Source: CAD feature listing. Evaluate the final solid. Frame: model axes, mm. Face numbers are marked on the shaded views. A direction names the side the tool comes from. Round coordinates to 2 decimals unless told otherwise and drop trailing zeros. Order: outer loops, then holes, each group sorted by start corner. A loop starts at its lowest first (then second) coordinate and runs counter-clockwise, first axis right, second up. Notation, with made-up numbers: (45.25, 1.25) -> (61.25, 1.25) arc R23 cw to (61.25, 14.25) -> close; hole circle Ø6 at (54.5, 48.25). An arc over 180 degrees is marked (long way). Answer as CSV lines item,"result".
Autodesk Fusion 360 part; units mm, degrees
sketch "Sketch1" plane through (0, 0, 0) normal (0, 0, 1) x (1, 0, 0)
  line L0 (-125, 90) -> (125, 90)
  line L1 (125, 90) -> (125, -90)
  line L2 (125, -90) -> (-125, -90)
  line L3 (-125, -90) -> (-125, 90)
  dimension "d1" = 250
  dimension "d2" = 180
  dimension "d3" = 90
  dimension "d4" = 125
extrude "Extrude1" add sketch "Sketch1" along normal blind 60
shell "Shell1" thickness 3 removed faces 1 at (-41.6667, 30, 60)
sketch "Sketch2" plane through (0, -90, 0) normal (0, -1, 0) x (1, 0, 0)
  line L0 (-125, 0) -> (125, 0)
  line L1 (125, 0) -> (125, 60)
  line L2 (125, 60) -> (-125, 60)
  line L3 (-125, 60) -> (-125, 0)
  circle A0 centre (-85, 30) radius 5
  circle A1 centre (25, 30) radius 5
  line L4 (-40, 35) -> (-10, 35)
  line L5 (-10, 35) -> (-10, 25)
  line L6 (-10, 25) -> (-40, 25)
  line L7 (-40, 25) -> (-40, 35)
  circle A2 centre (-110, 30) radius 6
  dimension "d8" = 10
  dimension "d9" = 10
  dimension "d10" = 12
extrude "Extrude2" cut sketch "Sketch2" against normal blind 10 contours A0 | A1 | L4 L5 L6 L7 | A2
sketch "Sketch3" plane through (0, 90, 0) normal (0, 1, 0) x (-1, 0, 0)
  line L0 (-125, 0) -> (125, 0)
  line L1 (125, 0) -> (125, 60)
  line L2 (125, 60) -> (-125, 60)
  line L3 (-125, 60) -> (-125, 0)
  circle A0 centre (105, 40) radius 5
  circle A1 centre (105, 25) radius 5
  circle A2 centre (90, 25) radius 5
  circle A3 centre (90, 40) radius 5
  circle A4 centre (105, 25) radius 5
  circle A5 centre (60, 25) radius 5
  circle A6 centre (75, 25) radius 5
  circle A7 centre (75, 25) radius 5
  circle A8 centre (75, 40) radius 5
  circle A9 centre (60, 40) radius 5
  line L4 (35, 45) -> (45, 45)
  line L5 (45, 45) -> (45, 30)
  line L6 (45, 30) -> (35, 30)
  line L7 (35, 30) -> (35, 45)
  line L8 (-110, 49) -> (-75, 49)
  line L9 (-75, 49) -> (-75, 14)
  line L10 (-75, 14) -> (-110, 14)
  line L11 (-110, 14) -> (-110, 49)
  dimension "d13" = 10
  dimension "d14" = 10
  dimension "d15" = 10
  dimension "d16" = 10
  dimension "d17" = 10
  dimension "d18" = 10
  dimension "d19" = 10
  dimension "d20" = 10
  dimension "d21" = 10
  dimension "d22" = 10
extrude "Extrude3" cut sketch "Sketch3" against normal blind 10 contours A0 | A1 A4 | A2 | A3 | A5 | A6 A7 | A8 | A9 | L4 L5 L6 L7 | L8 L9 L10 L11
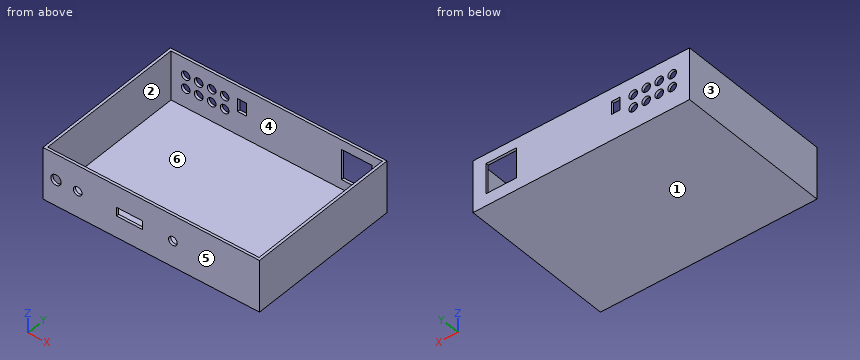
1. Mould query, pull axis X, two halves, no side actions, for the marked faces 1, 2, 3 and 4. Classes: released by +X, released by -X, zero draft, split by the parting line, or undercut.
Results below:
face 1,"zero draft"
face 2,"undercut"
face 3,"released by -X"
face 4,"undercut"
2. Reachability of the marked faces 5 and 6 from +Z, -Z, +X, -X, +Y, -Y: full face, straight path, thin tool, end or side. Return the list, or none.
Results below:
face 5,"+Z, -Z, +X, -X, -Y"
face 6,"+Z"
3. Pin query (flat end, axial travel): pin 1 (9 mm diameter, centred on x = -90, z = 25, fed in from +Y). Return the tip coordinate at first contact, or that it passes through.
Results below:
pin 1,"y = -87"
4. Section query A-A on x = 25. Return loops of the section in (y, z).
Results below:
outline,"(-90, 0) -> (90, 0) -> (90, 60) -> (87, 60) -> (87, 3) -> (-87, 3) -> (-87, 25) -> (-90, 25) -> close; (-90, 35) -> (-87, 35) -> (-87, 60) -> (-90, 60) -> close"
5. Section query B-B on z = 40. Give the number of separate pieces and of enclosed holes in the cut face, and give its area (3 significant figures).
Results below:
separate pieces,"6"
enclosed holes,"0"
area,"2,290 mm2"
6. Line query: L1, parallel to Z at x = -75, y = 88; L2, parallel to X at y = 55, z = 8.5; L3, parallel to Y at x = -48.5, z = 23.5. Output: solid intervals per line, ascending. Write a range as [from, to].
Results below:
L1,"[0, 20], [30, 35], [45, 60]"
L2,"[-125, -122], [122, 125]"
L3,"[-90, -87], [87, 90]"
7. Section query C-C on y = -47. Return loops of the section in (x, z).
Results below:
outline,"(-125, 0) -> (125, 0) -> (125, 60) -> (122, 60) -> (122, 3) -> (-122, 3) -> (-122, 60) -> (-125, 60) -> close"
